Source: three-view drawing plus pictorial views. Frame: mm from the lowest corner of the part. Coordinates: 2 decimals unless noted, no trailing zeros. Order: outer loops, then holes, each group sorted by start corner. A loop starts at its lowest first (then second) coordinate and runs counter-clockwise, first axis right, second up. Notation, with made-up numbers: (8, 46.5) - (12, 46.5) arc R19 ccw to (12, 82.5) - close; hole circle Ø3 at (41, 57.25). An arc over 180 degrees is marked (long way). One line per question, with ' | ' between items.
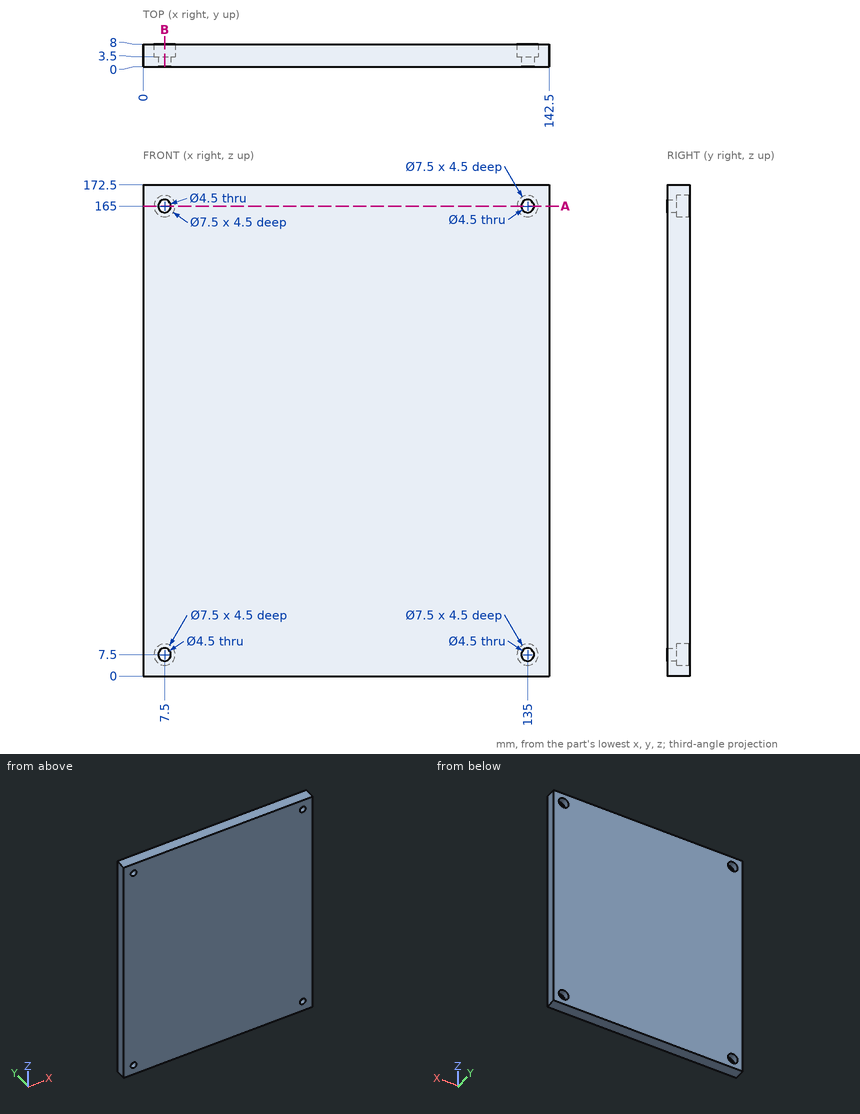
Item 1: Section A-A on z = 165. Return the cut outline in (x, y), and give its area (3 significant figures).
Data:
outline: (0, 0) - (5.25, 0) - (5.25, 3.5) - (3.75, 3.5) - (3.75, 8) - (0, 8) - close; (9.75, 0) - (132.75, 0) - (132.75, 3.5) - (131.25, 3.5) - (131.25, 8) - (11.25, 8) - (11.25, 3.5) - (9.75, 3.5) - close; (137.25, 0) - (142.5, 0) - (142.5, 8) - (138.75, 8) - (138.75, 3.5) - (137.25, 3.5) - close | area: 1,040 mm^2
Item 2: Section B-B on x = 7.5. Return the cut outline in (y, z).
Data:
outline: (0, 0) - (8, 0) - (8, 3.75) - (3.5, 3.75) - (3.5, 5.25) - (0, 5.25) - close; (0, 9.75) - (3.5, 9.75) - (3.5, 11.25) - (8, 11.25) - (8, 161.25) - (3.5, 161.25) - (3.5, 162.75) - (0, 162.75) - close; (0, 167.25) - (3.5, 167.25) - (3.5, 168.75) - (8, 168.75) - (8, 172.5) - (0, 172.5) - close
Item 3: Contact query for a flat-ended pin moving along its axis: P1, Ø6, axis at x = 8, z = 7.5, coming from the +Y side. Output: stop coordinate, or through.
Data:
P1: y = 3.5
Item 4: Ray query, line 1 (X direction, y = 0.85, z = 7.5); line 2 (Z direction, x = 135, y = 2.8); line 3 (Z direction, x = 135, y = 5.3). Return the intervals inside material, ascending.
Data:
line 1: 0 to 5.25, 9.75 to 132.75, 137.25 to 142.5 | line 2: 0 to 5.25, 9.75 to 162.75, 167.25 to 172.5 | line 3: 0 to 3.75, 11.25 to 161.25, 168.75 to 172.5
